```python
from build123d import *

# Parameters (mm, degrees)
SKETCH1_R           = 3.175
BOSS_EXTRUDE1_DEPTH = 45.12
SKETCH2_W           = 6.35
SKETCH2_H           = 5.59727822
CUT_EXTRUDE1_DEPTH  = 7
SKETCH3_R           = 1.5
CUT_EXTRUDE2_DEPTH  = 7


with BuildPart() as part:
    # Sketch1 → Boss-Extrude1 (new body)
    with BuildSketch(Plane.XY):
        Circle(SKETCH1_R)
    extrude(amount=BOSS_EXTRUDE1_DEPTH)

    # Sketch2 → Cut-Extrude1 (cut)
    with BuildSketch(Plane(origin=(0, 0, 0), x_dir=(1, 0, 0), z_dir=(0, 1, 0))):
        with Locations((0, -2.79863911)):
            Rectangle(SKETCH2_W, SKETCH2_H)
    extrude(amount=-CUT_EXTRUDE1_DEPTH, mode=Mode.SUBTRACT)

    # Sketch3 → Cut-Extrude2 (cut)
    with BuildSketch(Plane.XZ):
        with Locations((0, 2.79863911)):
            Circle(SKETCH3_R)
    extrude(amount=-CUT_EXTRUDE2_DEPTH, mode=Mode.SUBTRACT)


solid = part.part
```
Build history of the part. All positions in model axes, mm. A direction names the side the tool comes from. Round coordinates to 2 decimals unless told otherwise and drop trailing zeros. Loops run counter-clockwise (first coordinate to the right, second up) from the corner with the lowest first, then second, coordinate; pieces in that order, holes last.
Item 1: Saw through at B-B (y = 1.5). List the corners of the cut face in (x, z).
Item 2: Saw through at C-C (z = 36.5). List the corners of the cut face in (x, y) (3 decimals).
Item 3: Which spindle directions (+Z, -Z, +X, -X, +Y, -Y) get a long thin tool onto all of the face, cutting with end or side? Do faces 1 (the face through (0, 1, 0)), 2 (the face through (-1.5, 0, 2.1)). Say none if no direction does.
Item 4: Drill centre lines: line 1 along Z through (x, y) = (0, 1.95); line 2 along Y through (x, z) = (0.25, 29.5); line 3 along Z through (x, y) = (1.5, -2.5). Where is each one in solid material? Low to high.
Item 5: Two-plate mould, pull along X, no slides. Class faces 3 (the face through (1.386, 1.567, 2.224)), 4 (the face through (-0.41, 3.15, 22.24)), 5 (the face through (0, 0, 45.12)): released by +X, released by -X, zero draft, split by the parting line, or undercut.
Item 6: Pin check, flat tips, straight feed: P1, Ø1, axis at x = 1, z = 32, coming from the +Y side; P2, Ø2.5, axis at x = 0, z = 2.8, coming from the -Y side. Stop position of each tip, or through.
Item 7: Saw through at D-D (y = -1.75). List the corners of the cut face in (x, z).
Item 8: Saw through at A-A (x = 0). List the corners of the cut face in (y, z) (3 decimals).
Worked answers:
1. outline: (-2.8, 0) - (2.8, 0) - (2.8, 45.12) - (-2.8, 45.12) - close; hole circle Ø3 at (0, 2.8)
2. outline: circle Ø6.35 at (0, 0)
3. face 1: -Z, +X, -X, +Y, -Y
3. face 2: -Z, +X, -X, -Y
4. line 1: z = 0 to 1.3, 4.3 to 45.12
4. line 2: y = -3.17 to 3.17
4. line 3: z = 5.6 to 45.12
5. face 3: undercut
5. face 4: split by the parting line
5. face 5: zero draft
6. P1: stops at y = 3.14
6. P2: passes through
7. outline: (-2.65, 5.6) - (2.65, 5.6) - (2.65, 45.12) - (-2.65, 45.12) - close
8. outline: (-3.175, 5.597) - (0, 5.597) - (0, 4.299) - (3.175, 4.299) - (3.175, 45.12) - (-3.175, 45.12) - close; (0, 0) - (3.175, 0) - (3.175, 1.299) - (0, 1.299) - close
